Geometry check sheet. Reference: the model listing, model coordinates, mm. Face numbers are marked on the shaded views. Round coordinates to 2 decimals unless told otherwise and drop trailing zeros. Loops run counter-clockwise (first coordinate to the right, second up) from the corner with the lowest first, then second, coordinate; pieces in that order, holes last. Notation, with made-up numbers: (57, -32) - (65, -32) arc R15 cw to (65, -8) - close; hole circle Ø3 at (-16.5, 19). An arc over 180 degrees is marked (long way). Write item = value, one per line.
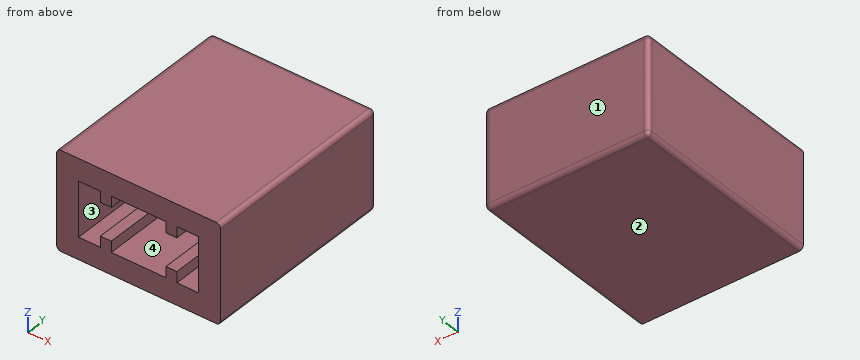
Autodesk Inventor part; units mm, degrees
ref_plane "YZ Plane" through (0, 0, 0) normal (1, 0, 0) x (0, 1, 0)
ref_plane "XZ Plane" through (0, 0, 0) normal (0, 1, 0) x (-1, 0, 0)
ref_plane "XY Plane" through (0, 0, 0) normal (0, 0, 1) x (1, 0, 0)
sketch "Náčrt1" plane through (0, 0, 0) normal (0, 1, 0) x (-1, 0, 0)
  line L0 (0, 0) -> (9.525, 0)
  line L1 (9.525, 0) -> (9.525, -5.715)
  line L2 (9.525, -5.715) -> (0, -5.715)
  line L3 (0, -5.715) -> (0, 0)
  dimension "d0" = 9.525
  dimension "d1" = 5.715
extrude "Vysunutí1" add sketch "Náčrt1" along normal blind 11.43
sketch "Náčrt2" plane through (0, 0, 0) normal (0, -1, 0) x (1, 0, 0)
  line L0 (-1.27, -4.445) -> (-1.27, -1.27)
  line L1 (-8.255, -1.27) -> (-8.255, -4.445)
  line L2 (-6.35, -4.445) -> (-3.175, -4.445)
  line L3 (-3.175, -1.27) -> (-6.35, -1.27)
  line L4 (-2.54, -1.27) -> (-2.54, -1.905)
  line L5 (-2.54, -1.905) -> (-3.175, -1.905)
  line L6 (-3.175, -1.905) -> (-3.175, -1.27)
  line L7 (-2.54, -4.445) -> (-2.54, -3.81)
  line L8 (-2.54, -3.81) -> (-3.175, -3.81)
  line L9 (-3.175, -3.81) -> (-3.175, -4.445)
  line L10 (-6.985, -4.445) -> (-6.985, -3.81)
  line L11 (-6.985, -3.81) -> (-6.35, -3.81)
  line L12 (-6.35, -3.81) -> (-6.35, -4.445)
  line L13 (-6.985, -1.27) -> (-6.985, -1.905)
  line L14 (-6.985, -1.905) -> (-6.35, -1.905)
  line L15 (-6.35, -1.905) -> (-6.35, -1.27)
  line L16 (-6.985, -1.27) -> (-8.255, -1.27)
  line L17 (-8.255, -4.445) -> (-6.985, -4.445)
  line L18 (-6.35, -4.445) -> (-3.175, -4.445)
  line L19 (-2.54, -4.445) -> (-1.27, -4.445)
  line L20 (-1.27, -1.27) -> (-2.54, -1.27)
  line L21 (-3.175, -1.27) -> (-6.35, -1.27)
  point P0 (-4.7625, -2.8575)
extrude "Vysunutí2" cut sketch "Náčrt2" against normal blind 9.525
fillet "Zaoblení1" radius 0.254 8 edges at (-4.7625, 11.43, 0) (-9.525, 5.715, 0) (-9.525, 11.43, -2.8575) (0, 11.43, -2.8575) (-4.7625, 11.43, -5.715) (-9.525, 5.715, -5.715) (0, 5.715, 0) (0, 5.715, -5.715)
properties part number "Button"
(1) Scan lines: L1, parallel to X at y = 7, z = -4.3 (3 decimals); L2, parallel to Z at x = -8, y = 2 (3 decimals); L3, parallel to Z at x = -6.5, y = 3.25 (3 decimals). Record each from-to range of solid material in increasing order. Write a range as [from, to].
Answers follow:
L1 = [-9.525, -8.255], [-6.985, -6.35], [-3.175, -2.54], [-1.27, 0]
L2 = [-5.715, -4.445], [-1.27, 0]
L3 = [-5.715, -3.81], [-1.905, 0]
(2) Section check B-B (z = -1.55). Enter the section's corners in (x, y) (3 decimals), then the cut area to 3 significant figures.
Answers follow:
outline = (-9.525, 0) - (-8.255, 0) - (-8.255, 9.525) - (-6.985, 9.525) - (-6.985, 0) - (-6.35, 0) - (-6.35, 9.525) - (-3.175, 9.525) - (-3.175, 0) - (-2.54, 0) - (-2.54, 9.525) - (-1.27, 9.525) - (-1.27, 0) - (0, 0) - (0, 11.176) arc R0.254 ccw to (-0.254, 11.43) - (-9.271, 11.43) arc R0.254 ccw to (-9.525, 11.176) - close
area = 54.4 mm²
(3) Section check C-C (x = -6.5). Enter the section's corners in (y, z) (3 decimals).
Answers follow:
outline = (0, -5.715) - (11.176, -5.715) arc R0.254 ccw to (11.43, -5.461) - (11.43, -0.254) arc R0.254 ccw to (11.176, 0) - (0, 0) - (0, -1.905) - (9.525, -1.905) - (9.525, -3.81) - (0, -3.81) - close
(4) Mould release check, pull along Z, two halves, no side actions. Record for the marked faces 1, 2, 3 and 4: pulls with the +Z half, pulls with the -Z half, needs draft (parallel to the pull), parting line crosses it, or undercut.
Answers follow:
face_1 = needs draft
face_2 = pulls with the -Z half
face_3 = undercut
face_4 = undercut
(5) Section check A-A (y = 2.25). Enter the section's corners in (x, z) (3 decimals).
Answers follow:
outline = (-9.525, -5.461) arc R0.254 ccw to (-9.271, -5.715) - (-0.254, -5.715) arc R0.254 ccw to (0, -5.461) - (0, -0.254) arc R0.254 ccw to (-0.254, 0) - (-9.271, 0) arc R0.254 ccw to (-9.525, -0.254) - close; hole (-8.255, -4.445) - (-6.985, -4.445) - (-6.985, -3.81) - (-6.35, -3.81) - (-6.35, -4.445) - (-3.175, -4.445) - (-3.175, -3.81) - (-2.54, -3.81) - (-2.54, -4.445) - (-1.27, -4.445) - (-1.27, -1.27) - (-2.54, -1.27) - (-2.54, -1.905) - (-3.175, -1.905) - (-3.175, -1.27) - (-6.35, -1.27) - (-6.35, -1.905) - (-6.985, -1.905) - (-6.985, -1.27) - (-8.255, -1.27) - close
(6) Section check D-D (x = -4.5). Enter the section's corners in (y, z) (3 decimals).
Answers follow:
outline = (0, -5.715) - (11.176, -5.715) arc R0.254 ccw to (11.43, -5.461) - (11.43, -0.254) arc R0.254 ccw to (11.176, 0) - (0, 0) - (0, -1.27) - (9.525, -1.27) - (9.525, -4.445) - (0, -4.445) - close
